Here's how the part is built. I have some questions about the finished solid (model axes, mm). Face numbers are marked on the shaded views. A direction names the side the tool comes from. Give positions to 0.01 mm unless a question says otherwise; leave off trailing zeros. Loops run counter-clockwise (first coordinate to the right, second up) from the corner with the lowest first, then second, coordinate; pieces in that order, holes last. Notation, with made-up numbers: (86, 88.25) -> (102, 88.25) arc R28 ccw to (102, 112.25) -> close; hole circle Ø6 at (-17.5, 0). An arc over 180 degrees is marked (long way). Answer in a Markdown table with one row per item. Add a question column.
Item 1: If we section it at B-B (z = -0.5): Write out the boundary of the cut face in (x, y), then the cut area to 3 significant figures.
Item 2: We'd pull the mould along Y, two halves only. Please class the marked faces 3, 4 and 5: released by +Y, released by -Y, zero draft, split by the parting line, or undercut.
Item 3: If we section it at A-A (x = 0): Write out the boundary of the cut face in (y, z), then the cut area to 3 significant figures.
Item 4: For P1, Ø5, axis at x = -1.5, y = -3.5, coming from the +Z side; P2, Ø6, axis at x = 6, y = 4, coming from the +Z side, each with a flat end and sliding along its axis, tell me the tip position at first contact or that it passes through.
Item 5: Which directions (+Z, -Z, +X, -X, +Y, -Y) give clear straight access to the entire face, cutting with the end or side of a thin tool? Please do the marked faces 1 and 2.
Item 6: If we section it at D-D (z = -8.25): Write out the boundary of the cut face in (x, y), then the cut area to 3 significant figures.
Item 7: If we section it at C-C (y = -4): Write out the boundary of the cut face in (x, z), then the cut area to 3 significant figures.
Item 8: If I drill on line 1 (Y direction, x = -7, z = -3); line 2 (Y direction, x = 0, z = 0.65), over which ranges is the centre line in solid material (lowest first)?
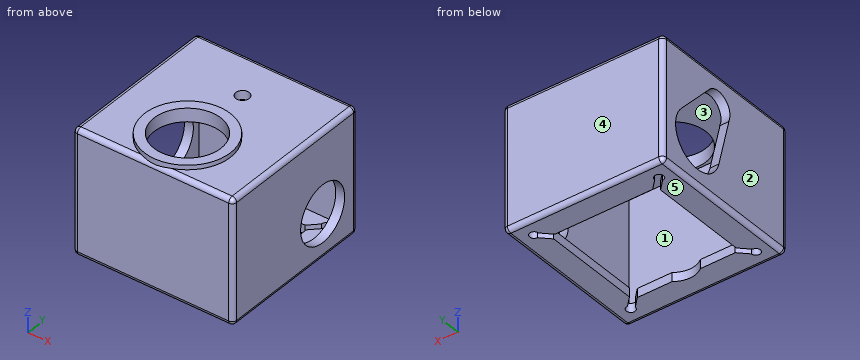
Autodesk Inventor part; units mm, degrees
ref_plane "YZ Plane" through (0, 0, 0) normal (1, 0, 0) x (0, 1, 0)
ref_plane "XZ Plane" through (0, 0, 0) normal (0, 1, 0) x (-1, 0, 0)
ref_plane "XY Plane" through (0, 0, 0) normal (0, 0, 1) x (1, 0, 0)
sketch "Эскиз1" plane through (0, 0, 0) normal (0, 0, 1) x (1, 0, 0)
  line L0 (-8, -8) -> (8, -8)
  line L1 (8, -8) -> (8, 8)
  line L2 (8, 8) -> (-8, 8)
  line L3 (-8, 8) -> (-8, -8)
  circle A0 centre (0, -4) radius 2.3157
  circle A1 centre (0, 4) radius 0.75
  line L4 (-9, -9) -> (9, -9)
  line L5 (9, -9) -> (9, 9)
  line L6 (9, 9) -> (-9, 9)
  line L7 (-9, 9) -> (-9, -9)
  point P0 (0, 0)
  dimension "d0" = 16
  dimension "d1" = 16
  dimension "d2" = 8
  dimension "d3" = 8
  dimension "d4" = 1.5
  dimension "d5" = 4
  dimension "d6" = 4
  dimension "d7" = 1
extrude "Выдавливание1" add sketch "Эскиз1" along normal blind 1 contours L3 L2 L1 L0 | L7 L6 L5 L4
extrude "Выдавливание2" add sketch "Эскиз1" against normal blind 13 contours L7 L6 L5 L4
sketch "Эскиз2" plane through (0, 0, -13) normal (0, 0, -1) x (-1, 0, 0)
  line L0 (-8, -8) -> (-8, 8)
  line L1 (-8, 8) -> (8, 8)
  line L2 (8, 8) -> (8, -8)
  line L3 (8, -8) -> (-8, -8)
  line L4 (-9, -9) -> (9, -9)
  line L5 (9, -9) -> (9, 9)
  line L6 (9, 9) -> (-9, 9)
  line L7 (-9, 9) -> (-9, -9)
  line L8 (-6, 5.5) -> (-6, -5.5)
  line L9 (6, -5.5) -> (6, 5.5)
  line L10 (5.5, 6) -> (-5.5, 6)
  spline S0 degree 3 number of poles 196 construction
  circle A0 centre (0, -4) radius 2.3157
  arc A1 (-1.5842, -6) -> (1.5842, -6) centre (0, -4) ccw
  line L11 (-5.5, -6) -> (-1.5842, -6)
  line L12 (-1.1537, -6) -> (-1.1341, -6)
  line L13 (1.5842, -6) -> (5.5, -6)
  line L14 (1.1397, -6) -> (1.1535, -6)
  line L15 (-8, -8) -> (8, -8) construction
  line L16 (-8, -8) -> (8, 8) construction
  line L17 (8, 8) -> (-8, 8) construction
  line L18 (-8, 8) -> (8, -8) construction
  line L19 (7.0273, 7.0273) -> (-7.0273, 7.0273) construction
  line L20 (-7.0273, 7.0273) -> (-7.0273, -7.0273) construction
  line L21 (-7.0273, -7.0273) -> (7.0273, -7.0273) construction
  line L22 (7.0273, -7.0273) -> (7.0273, 7.0273) construction
  line L23 (7.0273, 7.0273) -> (-7.0273, -7.0273) construction
  line L24 (-7.0273, 7.0273) -> (7.0273, -7.0273) construction
  arc A2 (-7.0273, -6.5273) -> (-6.5273, -7.0273) centre (-7.0273, -7.0273) ccw
  arc A3 (-6.5273, 7.0273) -> (-7.0273, 6.5273) centre (-7.0273, 7.0273) ccw
  arc A4 (7.0273, 6.5273) -> (6.5273, 7.0273) centre (7.0273, 7.0273) ccw
  arc A5 (6.5273, -7.0273) -> (7.0273, -6.5273) centre (7.0273, -7.0273) ccw
  line L25 (-6, -5.5) -> (-7.0273, -6.5273)
  line L26 (-6.5273, -7.0273) -> (-5.5, -6)
  line L27 (-6, 5.5) -> (-7.0273, 6.5273)
  line L28 (-6.5273, 7.0273) -> (-5.5, 6)
  line L29 (6.5273, -7.0273) -> (5.5, -6)
  line L30 (0, -0.5) -> (-0.5, 0)
  line L31 (0, 0.5) -> (0.5, 0)
  line L32 (6, -5.5) -> (7.0273, -6.5273)
  line L33 (0, -0.5) -> (0.5, 0)
  line L34 (6, 5.5) -> (7.0273, 6.5273)
  line L35 (6.5273, 7.0273) -> (5.5, 6)
  line L36 (0, 0.5) -> (-0.5, 0)
  point P0 (0, 0)
  dimension "d12" = 2
  dimension "d16" = 1
  dimension "d17" = 1
  dimension "d18" = 1
  dimension "d19" = 1
extrude "Выдавливание3" add sketch "Эскиз2" against normal blind 1 contours L0 L1 L2 L3
fillet "Сопряжение1" radius 0.5 12 edges at (9, -9, -6) (-9, -9, -6) (-9, 9, -6) (9, 9, -6) (-9, 0, 1) (0, -9, 1) (0, 9, 1) (9, 0, 1) (0, 9, -13) (9, 0, -13) (0, -9, -13) (-9, 0, -13)
sketch "Эскиз3" plane through (0, 0, 1) normal (0, 0, 1) x (1, 0, 0)
  circle A0 centre (0, -4) radius 2.3157
  circle A1 centre (0, -4) radius 2.3157
  circle A2 centre (0, -4) radius 3.75
  circle A3 centre (0, -4) radius 4.8299
  point P0 (0, 0)
  dimension "d22" = 7.5
extrude "Выдавливание4" add sketch "Эскиз3" along normal mid plane 1 contours A3
extrude "Выдавливание5" cut sketch "Эскиз3" against normal blind 1 contours A2
sketch "Эскиз4" plane through (-9, -8.5, 0.5) normal (-1, 0, 0) x (0, 0, 1)
  circle A0 centre (-8.5, 12.5) radius 3.2
  circle A1 centre (-3, 9.5) radius 1.7
  line L0 (-3.8644, 8.0362) -> (-3.6612, 7.9162)
  line L1 (-3.6612, 7.9162) -> (-9.3151, 9.4056)
  line L2 (-1.8523, 10.7541) -> (-6.3396, 14.8607)
  point P0 (-0.5, 8.5)
extrude "Выдавливание6" cut sketch "Эскиз4" against normal blind 20 contours A0
extrude "Выдавливание7" cut sketch "Эскиз4" against normal blind 2
properties part number "кожух  блока"
Recorded:
| question | item | result |
|---|---|---|
| 1 | outline | (-9, -8.5) arc R0.5 ccw to (-8.5, -9) -> (8.5, -9) arc R0.5 ccw to (9, -8.5) -> (9, 8.5) arc R0.5 ccw to (8.5, 9) -> (-8.5, 9) arc R0.5 ccw to (-9, 8.5) -> close; hole (-8, -8) -> (8, -8) -> (8, 8) -> (-8, 8) -> close |
| 1 | area | 67.8 mm^2 |
| 2 | face 3 | undercut |
| 2 | face 4 | released by +Y |
| 2 | face 5 | zero draft |
| 3 | outline | (-9, -12.5) arc R0.5 ccw to (-8.5, -13) -> (-6.55, -13) -> (-6.55, -12) -> (-8, -12) -> (-8, 0) -> (-7.75, 0) -> (-7.75, 1.5) -> (-8.83, 1.5) -> (-8.83, 0.88) arc R0.5 ccw to (-9, 0.5) -> close; (-0.25, 0) -> (3.25, 0) -> (3.25, 1) -> (0.83, 1) -> (0.83, 1.5) -> (-0.25, 1.5) -> close; (4.75, 0) -> (8, 0) -> (8, -12) -> (6, -12) -> (6, -13) -> (8.5, -13) arc R0.5 ccw to (9, -12.5) -> (9, 0.5) arc R0.5 ccw to (8.5, 1) -> (4.75, 1) -> close |
| 3 | area | 39.3 mm^2 |
| 4 | P1 | stops at z = 1.5 |
| 4 | P2 | stops at z = 1 |
| 5 | face 1 | none |
| 5 | face 2 | +Z, -Z, -X, +Y, -Y |
| 6 | outline | (-9, -8.5) arc R0.5 ccw to (-8.5, -9) -> (8.5, -9) arc R0.5 ccw to (9, -8.5) -> (9, 0.81) -> (8, 0.81) -> (8, -8) -> (-8, -8) -> (-8, 0.76) -> (-9, 0.76) -> close; (-9, 7.19) -> (-8, 7.19) -> (-8, 8) -> (8, 8) -> (8, 7.19) -> (9, 7.19) -> (9, 8.5) arc R0.5 ccw to (8.5, 9) -> (-8.5, 9) arc R0.5 ccw to (-9, 8.5) -> close |
| 6 | area | 55.0 mm^2 |
| 7 | outline | (-9, -12.5) arc R0.5 ccw to (-8.5, -13) -> (-6, -13) -> (-6, -12) -> (-8, -12) -> (-8, 0) -> (-3.75, 0) -> (-3.75, 1.5) -> (-4.83, 1.5) -> (-4.83, 1) -> (-8.5, 1) arc R0.5 ccw to (-9, 0.5) -> close; (3.75, 0) -> (8, 0) -> (8, -12) -> (6, -12) -> (6, -13) -> (8.5, -13) arc R0.5 ccw to (9, -12.5) -> (9, 0.5) arc R0.5 ccw to (8.5, 1) -> (4.83, 1) -> (4.83, 1.5) -> (3.75, 1.5) -> close |
| 7 | area | 41.4 mm^2 |
| 8 | line 1 | y = -9 to -8, 8 to 9 |
| 8 | line 2 | y = -8.98 to -7.75, -0.25 to 3.25, 4.75 to 8.98 |
